from build123d import *

# Parameters (mm, degrees)
F0_W     = 12.7
F0_H     = 9.525
F0_H_2   = 19.05
F1_DEPTH = 25.4
F2_W     = 25.4
F2_H     = 31.75
F3_DEPTH = 38.101
F5_DEPTH = 19.051
F7_DEPTH = 50.801


with BuildPart() as f1:
    # F0 (on Front) → F1 (new body, symmetric)
    with BuildSketch(Plane.XZ):
        with Locations((31.75, -14.2875)):
            Rectangle(F0_W, F0_H)
        with Locations((19.05, -14.2875)):
            Rectangle(F0_W, F0_H)
        with Locations((31.75, 0)):
            Rectangle(F0_W, F0_H_2)
        Polygon((-38.1, -19.05), (12.7, -19.05), (12.7, -9.525), (12.7, 9.525), (12.7, 19.05), (-38.1, 19.05), align=None)
        with Locations((31.75, 14.2875)):
            Rectangle(F0_W, F0_H)
        with Locations((19.05, 14.2875)):
            Rectangle(F0_W, F0_H)
        with Locations((19.05, 0)):
            Rectangle(F0_W, F0_H_2)
    extrude(amount=F1_DEPTH, both=True)

    # F2 (on face) → F3 (cut, through all)
    with BuildSketch(Plane.XY.offset(19.05)):
        with Locations((25.4, -9.525)):
            Rectangle(F2_W, F2_H)
    extrude(amount=-F3_DEPTH, mode=Mode.SUBTRACT)

    # F4 (on face) → F5 (cut, through all)
    with BuildSketch(Plane.XZ.offset(-6.35)):
        with BuildLine():
            ThreePointArc((31.9484375, 9.525), (30.0304445624, 14.1554445624), (25.4, 16.0734375))
            Line((25.4, 16.0734375), (25.4, 9.525))
            Line((25.4, 9.525), (31.9484375, 9.525))
        make_face()
        with BuildLine():
            ThreePointArc((31.9484375, -9.525), (30.0304445624, -4.8945554376), (25.4, -2.9765625))
            Line((25.4, -2.9765625), (25.4, -9.525))
            Line((25.4, -9.525), (31.9484375, -9.525))
        make_face()
        with BuildLine():
            Line((25.4, -9.525), (25.4, -2.9765625))
            ThreePointArc((25.4, -2.9765625), (20.7695554376, -4.8945554376), (18.8515625, -9.525))
            Line((18.8515625, -9.525), (25.4, -9.525))
        make_face()
        with BuildLine():
            Line((25.4, 9.525), (25.4, 16.0734375))
            ThreePointArc((25.4, 16.0734375), (20.7695554376, 14.1554445624), (18.8515625, 9.525))
            Line((18.8515625, 9.525), (25.4, 9.525))
        make_face()
        with BuildLine():
            Line((31.9484375, 9.525), (25.4, 9.525))
            Line((25.4, 9.525), (25.4, 2.9765625))
            ThreePointArc((25.4, 2.9765625), (30.0304445624, 4.8945554376), (31.9484375, 9.525))
        make_face()
        with BuildLine():
            Line((25.4, 2.9765625), (25.4, 9.525))
            Line((25.4, 9.525), (18.8515625, 9.525))
            ThreePointArc((18.8515625, 9.525), (20.7695554376, 4.8945554376), (25.4, 2.9765625))
        make_face()
        with BuildLine():
            Line((31.9484375, -9.525), (25.4, -9.525))
            Line((25.4, -9.525), (25.4, -16.0734375))
            ThreePointArc((25.4, -16.0734375), (30.0304445624, -14.1554445624), (31.9484375, -9.525))
        make_face()
        with BuildLine():
            Line((25.4, -16.0734375), (25.4, -9.525))
            Line((25.4, -9.525), (18.8515625, -9.525))
            ThreePointArc((18.8515625, -9.525), (20.7695554376, -14.1554445624), (25.4, -16.0734375))
        make_face()
    extrude(amount=-F5_DEPTH, mode=Mode.SUBTRACT)

    # F6 (on face) → F7 (cut, through all)
    with BuildSketch(Plane.YZ.offset(12.7)):
        with BuildLine():
            ThreePointArc((-3.175, 9.525), (-5.0348719395, 14.0151280605), (-9.525, 15.875))
            Line((-9.525, 15.875), (-9.525, 9.525))
            Line((-9.525, 9.525), (-3.175, 9.525))
        make_face()
        with BuildLine():
            ThreePointArc((-3.175, -9.525), (-5.0348719395, -5.0348719395), (-9.525, -3.175))
            Line((-9.525, -3.175), (-9.525, -9.525))
            Line((-9.525, -9.525), (-3.175, -9.525))
        make_face()
        with BuildLine():
            Line((-9.525, -9.525), (-9.525, -3.175))
            ThreePointArc((-9.525, -3.175), (-14.0151280605, -5.0348719395), (-15.875, -9.525))
            Line((-15.875, -9.525), (-9.525, -9.525))
        make_face()
        with BuildLine():
            Line((-9.525, 9.525), (-9.525, 15.875))
            ThreePointArc((-9.525, 15.875), (-14.0151280605, 14.0151280605), (-15.875, 9.525))
            Line((-15.875, 9.525), (-9.525, 9.525))
        make_face()
        with BuildLine():
            Line((-3.175, 9.525), (-9.525, 9.525))
            Line((-9.525, 9.525), (-9.525, 3.175))
            ThreePointArc((-9.525, 3.175), (-5.0348719395, 5.0348719395), (-3.175, 9.525))
        make_face()
        with BuildLine():
            Line((-9.525, 3.175), (-9.525, 9.525))
            Line((-9.525, 9.525), (-15.875, 9.525))
            ThreePointArc((-15.875, 9.525), (-14.0151280605, 5.0348719395), (-9.525, 3.175))
        make_face()
        with BuildLine():
            Line((-3.175, -9.525), (-9.525, -9.525))
            Line((-9.525, -9.525), (-9.525, -15.875))
            ThreePointArc((-9.525, -15.875), (-5.0348719395, -14.0151280605), (-3.175, -9.525))
        make_face()
        with BuildLine():
            Line((-9.525, -15.875), (-9.525, -9.525))
            Line((-9.525, -9.525), (-15.875, -9.525))
            ThreePointArc((-15.875, -9.525), (-14.0151280605, -14.0151280605), (-9.525, -15.875))
        make_face()
    extrude(amount=-F7_DEPTH, mode=Mode.SUBTRACT)


solid = f1.part
The listing builds one solid part. Answer for the finished solid, in the listing's coordinates (mm). A direction names the side the tool comes from. Coordinates: 2 decimals unless noted, no trailing zeros. Order: outer loops, then holes, each group sorted by start corner. A loop starts at its lowest first (then second) coordinate and runs counter-clockwise, first axis right, second up. Notation, with made-up numbers: (49.25, -20.5) -> (78.25, -20.5) arc R24 cw to (78.25, 8.5) -> close; hole circle Ø2 at (79, -5.75). An arc over 180 degrees is marked (long way). Answer in a Markdown table with one row per item. Add a question column.
Item 1: Find section C-C (z = -12.5). Write down the section's boundary in (x, y).
Item 2: Find the intervals of material crossed by L1, parallel to Z at x = -21.5, y = -10; L2, parallel to Z at x = 23, y = 21.5; L3, parallel to X at y = -23, z = 11, in increasing order. Write a range as from..to.
Item 3: Find section D-D (z = -0.5). Write down the section's boundary in (x, y), then the cut area to 3 significant figures.
Item 4: Which of the six approach directions +Z, -Z, +X, -X, +Y, -Y give full straight-line access (tool end or side, diameter ignored) to faces 1 (the face through (25, 6.35, 0)), 2 (the face through (-8, 0, 19.05))?
Item 5: Find section A-A (x = 5). Write down the section's boundary in (y, z) (3 decimals), then the cut area to 3 significant figures.
Item 6: Find section B-B (y = 21). Write down the section's boundary in (x, z) (3 decimals).
Item 7: Each of these flat-tipped pins is pushed along its axis until it touches: P1, Ø9.5, axis at y = -7, z = 1.5, coming from the +X side; P2, Ø3, axis at x = 22.5, z = 4, coming from the +Y side; P3, Ø20.5, axis at x = 31.5, z = -9, coming from the -Y side. Where does it stop, or does it pass through?
Result set:
| question | item | result |
|---|---|---|
| 1 | outline | (-38.1, -25.4) -> (12.7, -25.4) -> (12.7, -15.13) -> (-38.1, -15.13) -> close; (-38.1, -3.92) -> (12.7, -3.92) -> (12.7, 6.35) -> (19.57, 6.35) -> (19.57, 25.4) -> (-38.1, 25.4) -> close; (31.23, 6.35) -> (38.1, 6.35) -> (38.1, 25.4) -> (31.23, 25.4) -> close |
| 2 | L1 | z = -19.05..-15.86, -3.19..3.19, 15.86..19.05 |
| 2 | L2 | z = -19.05..-15.62, -3.43..3.43, 15.62..19.05 |
| 2 | L3 | x = -38.1..12.7 |
| 3 | outline | (-38.1, -25.4) -> (12.7, -25.4) -> (12.7, 6.35) -> (38.1, 6.35) -> (38.1, 25.4) -> (-38.1, 25.4) -> close |
| 3 | area | 3,060 mm² |
| 4 | face 1 | +Z, -Z, +X, -Y |
| 4 | face 2 | +Z, +X, -X, +Y, -Y |
| 5 | outline | (-25.4, -19.05) -> (25.4, -19.05) -> (25.4, 19.05) -> (-25.4, 19.05) -> close; hole circle Ø12.7 at (-9.525, -9.525); hole circle Ø12.7 at (-9.525, 9.525) |
| 5 | area | 1,680 mm² |
| 6 | outline | (-38.1, -19.05) -> (38.1, -19.05) -> (38.1, 19.05) -> (-38.1, 19.05) -> close; hole circle Ø13.097 at (25.4, -9.525); hole circle Ø13.097 at (25.4, 9.525) |
| 7 | P1 | stops at x = 12.7 |
| 7 | P2 | stops at y = 25.4 |
| 7 | P3 | stops at y = 6.35 |
